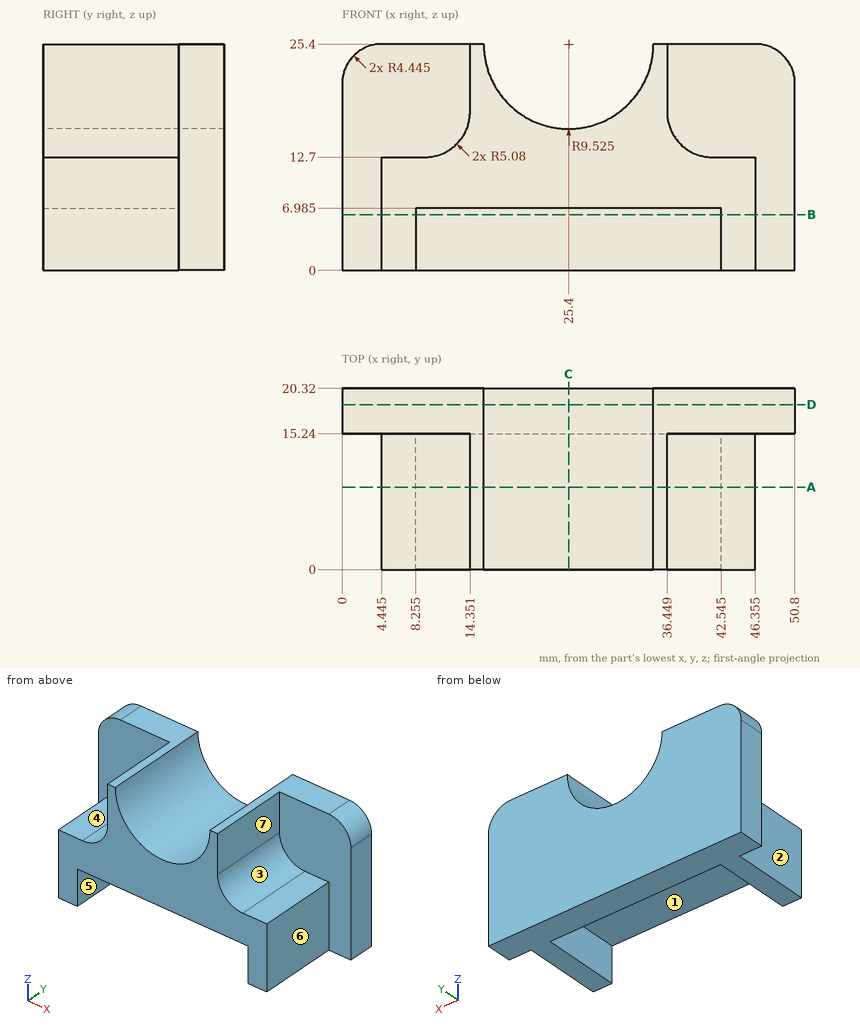
Print and shaded views of the part. All mm, measured from the part's lowest x, y and z. A direction names the side the tool comes from. Round coordinates to 2 decimals unless told otherwise and drop trailing zeros. Order: outer loops, then holes, each group sorted by start corner. A loop starts at its lowest first (then second) coordinate and runs counter-clockwise, first axis right, second up. Notation, with made-up numbers: (27.5, 86.5) - (66.5, 86.5) arc R10 ccw to (66.5, 105.5) - close; hole circle Ø8 at (-0.5, 8.25). An arc over 180 degrees is marked (long way). Use a Markdown table: item, result.
1) Tool access for the marked faces 4, 5, 6 and 7: list every direction of +Z, -Z, +X, -X, +Y, -Y with a clear straight run to the whole face (end or side of a thin tool).
Recorded:
| item | result |
|---|---|
| face 4 | +Z, -X, -Y |
| face 5 | -Z, -Y |
| face 6 | +Z, -Z, +X, -Y |
| face 7 | +Z, +X, -Y |
2) Saw through at A-A on y = 9.25. Write the cut outline in (x, z) (3 decimals).
Recorded:
| item | result |
|---|---|
| outline | (4.445, 0) - (8.255, 0) - (8.255, 6.985) - (42.545, 6.985) - (42.545, 0) - (46.355, 0) - (46.355, 12.7) - (41.529, 12.7) arc R5.08 cw to (36.449, 17.78) - (36.449, 25.4) - (34.925, 25.4) arc R9.525 cw to (15.875, 25.4) - (14.351, 25.4) - (14.351, 17.78) arc R5.08 cw to (9.271, 12.7) - (4.445, 12.7) - close |
3) Saw through at C-C on x = 25.4. Write the cut outline in (y, z) (3 decimals), and give its area (3 significant figures).
Recorded:
| item | result |
|---|---|
| outline | (0, 6.985) - (15.24, 6.985) - (15.24, 0) - (20.32, 0) - (20.32, 15.875) - (0, 15.875) - close |
| area | 216 mm² |
4) Saw through at B-B on z = 6.25. Write the cut outline in (x, y) (3 decimals), and give its area (3 significant figures).
Recorded:
| item | result |
|---|---|
| outline | (0, 15.24) - (4.445, 15.24) - (4.445, 0) - (8.255, 0) - (8.255, 15.24) - (42.545, 15.24) - (42.545, 0) - (46.355, 0) - (46.355, 15.24) - (50.8, 15.24) - (50.8, 20.32) - (0, 20.32) - close |
| area | 374 mm² |
5) Saw through at D-D on y = 18.5. Write the cut outline in (x, z) (3 decimals).
Recorded:
| item | result |
|---|---|
| outline | (0, 0) - (50.8, 0) - (50.8, 20.955) arc R4.445 ccw to (46.355, 25.4) - (34.925, 25.4) arc R9.525 cw to (15.875, 25.4) - (4.445, 25.4) arc R4.445 ccw to (0, 20.955) - close |
6) Flat gauge pins, fed straight in: pin 1 Ø10 at (x, y) = (36.5, 9.5) entering from +Z; pin 2 Ø10 at (y, z) = (7.5, 9) entering from +X (3 decimals); pin 3 Ø5 at (x, y) = (25.5, 15) entering from +Z; pin 4 Ø4 at (x, y) = (5.5, 11) entering from +Z. Where does each tip first touch, or does it go through?
Recorded:
| item | result |
|---|---|
| pin 1 | stops at z = 25.4 |
| pin 2 | stops at x = 46.355 |
| pin 3 | stops at z = 16.24 |
| pin 4 | stops at z = 12.7 |
7) Wall check: L1, parallel to X at y = 8.5, z = 5.5 (3 decimals); L2, parallel to Y at x = 3, z = 18; L3, parallel to Z at x = 44.5, y = 9.75. Give the ranges that are in metal, low to high.
Recorded:
| item | result |
|---|---|
| L1 | x = 4.445 to 8.255, 42.545 to 46.355 |
| L2 | y = 15.24 to 20.32 |
| L3 | z = 0 to 12.7 |
8) Pull direction X, two halves, no side cores. Call the marked faces 1, 2 and 3: pulls with the +X half, pulls with the -X half, needs draft (parallel to the pull), parting line crosses it, or undercut.
Recorded:
| item | result |
|---|---|
| face 1 | undercut |
| face 2 | pulls with the -X half |
| face 3 | pulls with the +X half |
